from build123d import *

# Parameters (mm, degrees)
SKETCH1_R           = 2
BOSS_EXTRUDE1_DEPTH = 2
SKETCH2_R           = 2.5
BOSS_EXTRUDE2_DEPTH = 35
FILLET1_R           = 2


with BuildPart() as part:
    # Sketch1 → Boss-Extrude1 (new body)
    with BuildSketch(Plane(origin=(0, 0, 0), x_dir=(1, 0, 0), z_dir=(0, 1, 0))):
        with BuildLine():
            Line((-65, 47), (-65, -47))
            Line((-65, -47), (-70, -52.103103631))
            Line((-70, -52.103103631), (-70, -72))
            ThreePointArc((-70, -72), (-68.535533906, -75.535533906), (-65, -77))
            Line((-65, -77), (65, -77))
            ThreePointArc((65, -77), (68.535533906, -75.535533906), (70, -72))
            Line((70, -72), (70, -52.103103631))
            Line((70, -52.103103631), (65, -47))
            Line((65, -47), (65, 47))
            Line((65, 47), (70, 51.898979486))
            Line((70, 51.898979486), (70, 72))
            ThreePointArc((70, 72), (68.535533906, 75.535533906), (65, 77))
            Line((65, 77), (-65, 77))
            ThreePointArc((-65, 77), (-68.535533906, 75.535533906), (-70, 72))
            Line((-70, 72), (-70, 51.898979486))
            Line((-70, 51.898979486), (-65, 47))
        make_face()
        with Locations(Location((-65, -72, 0), (0, 0, 270))):
            Circle(SKETCH1_R, mode=Mode.SUBTRACT)
        with Locations(Location((65, -72, 0), (0, 0, 270))):
            Circle(SKETCH1_R, mode=Mode.SUBTRACT)
        with Locations(Location((-65, 72, 0), (0, 0, 270))):
            Circle(SKETCH1_R, mode=Mode.SUBTRACT)
        with Locations(Location((65, 72, 0), (0, 0, 270))):
            Circle(SKETCH1_R, mode=Mode.SUBTRACT)
    extrude(amount=BOSS_EXTRUDE1_DEPTH)

    # Sketch2 → Boss-Extrude2 (add)
    with BuildSketch(Plane(origin=(0, 2, 0), x_dir=(1, 0, 0), z_dir=(0, 1, 0))):
        Polygon((-60, -24.852813742), (-24.852813742, -60.262270904), (24.852813742, -60.262270904), (60.262270904, -24.852813742), (60.262270904, 24.852813742), (24.852813742, 60.262270904), (-24.852813742, 60.262270904), (-60, 24.852813742), align=None)
        with Locations(Location((0, 0, 0), (0, 0, 270))):
            Circle(SKETCH2_R, mode=Mode.SUBTRACT)
    extrude(amount=BOSS_EXTRUDE2_DEPTH)

    # Fillet1
    fillet1_edges = [part.edges().sort_by_distance(p)[0] for p in [
        (-42.426406871, 37, -42.557542323),
        (-60, 37, 0),
        (-42.426406871, 37, 42.557542323),
        (0, 37, 60.262270904),
        (42.557542323, 37, 42.557542323),
        (60.262270904, 37, 0),
        (42.557542323, 37, -42.557542323),
        (0, 37, -60.262270904),
        (-42.426406871, 2, -42.557542323),
        (-24.852813742, 19.5, -60.262270904),
        (-60, 2, 0),
        (-60, 19.5, -24.852813742),
        (-42.426406871, 2, 42.557542323),
        (-60, 19.5, 24.852813742),
        (0, 2, 60.262270904),
        (-24.852813742, 19.5, 60.262270904),
        (42.557542323, 2, 42.557542323),
        (24.852813742, 19.5, 60.262270904),
        (60.262270904, 2, 0),
        (60.262270904, 19.5, 24.852813742),
        (42.557542323, 2, -42.557542323),
        (60.262270904, 19.5, -24.852813742),
        (0, 2, -60.262270904),
        (24.852813742, 19.5, -60.262270904),
    ]]
    fillet(fillet1_edges, radius=FILLET1_R)


solid = part.part
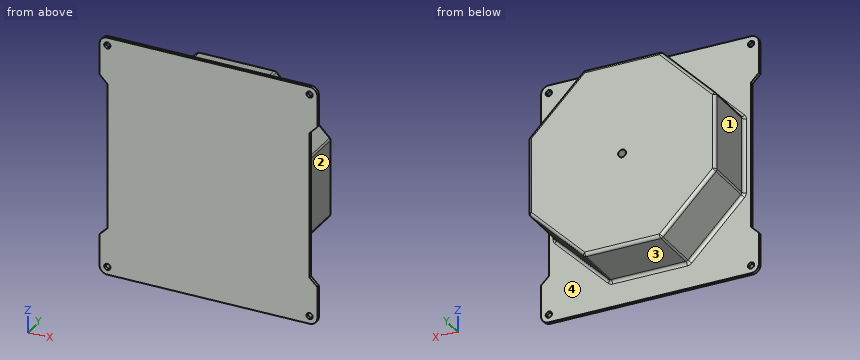
Read the model definition and answer for the solid it produces. Units are mm, in the model's axes. Face numbers are marked on the shaded views. A direction names the side the tool comes from. Round coordinates to 2 decimals unless told otherwise and drop trailing zeros. Loops run counter-clockwise (first coordinate to the right, second up) from the corner with the lowest first, then second, coordinate; pieces in that order, holes last.
Q1. Section C-C on x = 0 is taken. Write down the section's boundary in (y, z), and give its area (3 significant figures).
Q2. Section A-A on x = -20.5 is taken. Write down the section's boundary in (y, z).
Q3. Each of these flat-tipped pins is pushed along its axis until it touches: pin 1 (6 mm diameter, centred on x = -16, y = 19, fed in from +Z); pin 2 (4.5 mm diameter, centred on x = 65, z = -72, fed in from +Y); pin 3 (9.5 mm diameter, centred on y = 25.5, z = 9.5, fed in from +X). Where does it stop, or does it pass through?
Q4. Section B-B on y = 8.5 is taken. Write down the section's boundary in (x, z), and give its area (3 significant figures).
Q5. Which of the six approach directions +Z, -Z, +X, -X, +Y, -Y give full straight-line access (tool end or side, diameter ignored) to the marked faces 1, 2, 3 and 4?
Q6. Consider probe 1 along X at (y, z) = (0.7, -72); probe 2 along X at (y, z) = (30, 0); probe 3 along Z at (x, y) = (-21, 5). Determine where each line is inside the solid, lowest interval first.
Output:
1. outline: (0, -77) - (2, -77) - (2, -62.26) arc R2 cw to (4, -60.26) - (35, -60.26) arc R2 ccw to (37, -58.26) - (37, -2.5) - (2, -2.5) - (2, 2.5) - (37, 2.5) - (37, 58.26) arc R2 ccw to (35, 60.26) - (4, 60.26) arc R2 cw to (2, 62.26) - (2, 77) - (0, 77) - close
1. area: 4,350 mm2
2. outline: (0, -77) - (2, -77) - (2, -62.26) arc R2 cw to (4, -60.26) - (35, -60.26) arc R2 ccw to (37, -58.26) - (37, 58.26) arc R2 ccw to (35, 60.26) - (4, 60.26) arc R2 cw to (2, 62.26) - (2, 77) - (0, 77) - close
3. pin 1: stops at z = 60.26
3. pin 2: stops at y = 2
3. pin 3: stops at x = 60.26
4. outline: (-60, -24.03) arc R2 ccw to (-59.42, -25.44) - (-25.44, -59.67) arc R2 ccw to (-24.02, -60.26) - (24.02, -60.26) arc R2 ccw to (25.44, -59.68) - (59.68, -25.44) arc R2 ccw to (60.26, -24.02) - (60.26, 24.02) arc R2 ccw to (59.68, 25.44) - (25.44, 59.68) arc R2 ccw to (24.02, 60.26) - (-24.02, 60.26) arc R2 ccw to (-25.44, 59.67) - (-59.42, 25.44) arc R2 ccw to (-60, 24.03) - close; hole circle Ø5 at (0, 0)
4. area: 12,000 mm2
5. face 1: +Z, -Z, -X, +Y
5. face 2: +Z, -Z, +X, +Y
5. face 3: -Z, +X, -X, +Y
5. face 4: +Y
6. probe 1: x = -70 to -67, -63 to 63, 67 to 70
6. probe 2: x = -60 to -2.5, 2.5 to 60.26
6. probe 3: z = -60.26 to 60.26
